Geometry: final body of the model. Coordinates: model frame, mm. Face numbers are marked on the shaded views. A direction names the side the tool comes from. Give positions to 0.01 mm unless a question says otherwise; leave off trailing zeros. Loops run counter-clockwise (first coordinate to the right, second up) from the corner with the lowest first, then second, coordinate; pieces in that order, holes last. Notation, with made-up numbers: (53.5, 7.5) - (110.5, 7.5) arc R27 ccw to (110.5, 34.5) - close; hole circle Ø10 at (18, 46.25). An arc over 180 degrees is marked (long way). Answer in a Markdown table with one row per item.
from build123d import *

# Parameters (mm, degrees)
F0_W     = 150
F0_H     = 200
F1_DEPTH = 15
F2_R     = 60
F3_DEPTH = 81.44554


with BuildPart() as f1:
    # F0 (on Top) → F1 (new body)
    with BuildSketch(Plane.XY):
        with Locations((-6.63894, 50.128499)):
            Rectangle(F0_W, F0_H)
    extrude(amount=F1_DEPTH)

    # F2 (on Right) → F3 (join)
    with BuildSketch(Plane.YZ):
        with Locations((-4.760173, 7.580816)):
            Circle(F2_R)
    extrude(amount=F3_DEPTH)


solid = f1.part
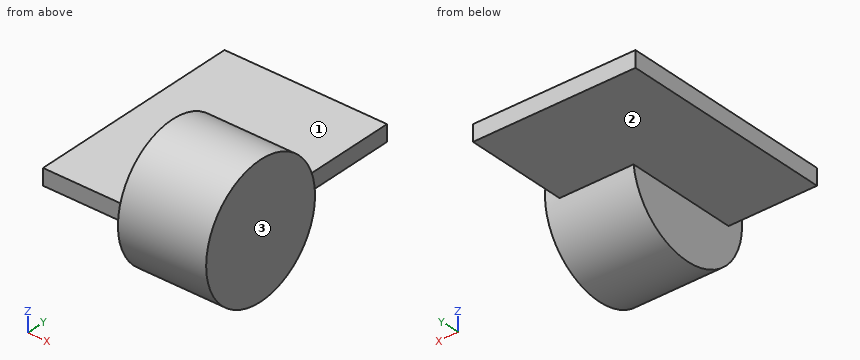
Q1. Cut plane C-C (z = 11.5). Output: boundary loops of the cut face in (x, y), and give its area (3 significant figures).
Check values:
| item | result |
|---|---|
| outline | (-81.64, -49.87) - (0, -49.87) - (0, -64.63) - (81.45, -64.63) - (81.45, 55.11) - (68.36, 55.11) - (68.36, 150.13) - (-81.64, 150.13) - close |
| area | 32,600 mm² |
Q2. First-contact query: pin 1 (4.5 mm diameter, centred on y = 94, z = 5.5, fed in from +X); pin 2 (4 mm diameter, centred on x = -57.5, y = 104.5, fed in from -Z); pin 3 (12 mm diameter, centred on x = -44, z = 6.5, fed in from -Y). Flat tips, straight axial feed; report the tip coordinate or a pass-through.
Check values:
| item | result |
|---|---|
| pin 1 | x = 68.36 |
| pin 2 | z = 0 |
| pin 3 | y = -49.87 |
Q3. Cut plane B-B (x = -22). Output: boundary loops of the cut face in (y, z), and give its area (3 significant figures).
Check values:
| item | result |
|---|---|
| outline | (-49.87, 0) - (150.13, 0) - (150.13, 15) - (-49.87, 15) - close |
| area | 3,000 mm² |
Q4. Cut plane A-A (y = -9). Output: boundary loops of the cut face in (x, z), and give its area (3 significant figures).
Check values:
| item | result |
|---|---|
| outline | (-81.64, 0) - (0, 0) - (0, -52.27) - (81.45, -52.27) - (81.45, 67.43) - (0, 67.43) - (0, 15) - (-81.64, 15) - close |
| area | 11,000 mm² |
Q5. Material intervals for line 1 along X through (y, z) = (93, 11); line 2 along Z through (x, y) = (-2.5, 52); line 3 along X through (y, z) = (-29.5, -37.5), sorted ascending.
Check values:
| item | result |
|---|---|
| line 1 | -81.64 to 68.36 |
| line 2 | 0 to 15 |
| line 3 | 0 to 81.45 |
Q6. Reachability of the marked faces 1, 2 and 3 from +Z, -Z, +X, -X, +Y, -Y: full face, straight path, thin tool, end or side. Return the list, or none.
Check values:
| item | result |
|---|---|
| face 1 | +Z, -X, +Y |
| face 2 | -Z, -X, +Y |
| face 3 | +Z, -Z, +X, +Y, -Y |
Q7. Cut plane D-D (x = 3). Output: boundary loops of the cut face in (y, z), and give its area (3 significant figures).
Check values:
| item | result |
|---|---|
| outline | (54.76, 0) - (150.13, 0) - (150.13, 15) - (54.78, 15) arc R60 ccw (long way) to start |
| area | 12,700 mm² |
